```python
from build123d import *

# Parameters (mm, degrees)
SKETCH_1_W          = 260
SKETCH_1_H          = 236
EXTRUDE_1_DEPTH     = 3
SKETCH_2_R          = 2.25
SKETCH_2_R_2        = 3.5
CUT_EXTRUDE_1_DEPTH = 4
SKETCH1_R           = 2.25
CUT_EXTRUDE1_DEPTH  = 4


with BuildPart() as part:
    # Эскиз1 → Бобышка-Вытянуть1 (new body)
    with BuildSketch(Plane.XZ):
        with Locations((-88.97919902, 98.072268451)):
            Rectangle(SKETCH_1_W, SKETCH_1_H)
    extrude(amount=EXTRUDE_1_DEPTH)

    # Эскиз2 → Вырез-Вытянуть1 (cut, through all)
    with BuildSketch(Plane.XZ.offset(3)):
        with Locations((-208.97919902, 98.072268451)):
            Circle(SKETCH_2_R)
        with Locations((-148.97919902, -9.927731549)):
            Circle(SKETCH_2_R)
        with Locations((-28.97919902, -9.927731549)):
            Circle(SKETCH_2_R)
        with Locations((31.02080098, 98.072268451)):
            Circle(SKETCH_2_R)
        with Locations((-28.97919902, 206.072268451)):
            Circle(SKETCH_2_R)
        with Locations((-148.97919902, 206.072268451)):
            Circle(SKETCH_2_R)
        with Locations((-208.97919902, -9.927731549)):
            Circle(SKETCH_2_R_2)
        with Locations((-208.97919902, 206.072268451)):
            Circle(SKETCH_2_R_2)
        with Locations((31.02080098, -9.927731549)):
            Circle(SKETCH_2_R_2)
        with Locations((31.02080098, 206.072268451)):
            Circle(SKETCH_2_R_2)
    extrude(amount=-CUT_EXTRUDE_1_DEPTH, mode=Mode.SUBTRACT)

    # Sketch1 → Cut-Extrude1 (cut, through all)
    with BuildSketch(Plane(origin=(0, 0, 0), x_dir=(1, 0, 0), z_dir=(0, 1, 0))):
        with Locations((-31.97919902, -141.072268451)):
            Circle(SKETCH1_R)
        with Locations((11.02080098, -98.072268451)):
            Circle(SKETCH1_R)
        with Locations((-31.97919902, -55.072268451)):
            Circle(SKETCH1_R)
    extrude(amount=-CUT_EXTRUDE1_DEPTH, mode=Mode.SUBTRACT)


solid = part.part
```
Check sheet for the modelled part. Datum: model origin and axes. Units: mm. Give positions to 0.01 mm unless a question says otherwise; leave off trailing zeros. Answer as CSV lines item,"result".
Item 1: Scan lines: L1, parallel to Z at x = -30, y = -1.05; L2, parallel to X at y = -2.4, z = 203.5; L3, parallel to X at y = -1.9, z = 99. Record each from-to range of solid material in increasing order.
Reply:
L1,"-19.93 to -11.93, -7.92 to 54, 56.14 to 140, 142.14 to 204.07, 208.08 to 216.07"
L2,"-218.98 to -211.35, -206.61 to 28.65, 33.39 to 41.02"
L3,"-218.98 to -211.03, -206.93 to 8.97, 13.07 to 28.97, 33.07 to 41.02"
Item 2: Depth check by flat-ended pin: pin 1 Ø4 at (x, z) = (-148.98, 206.07) entering from -Y; pin 2 Ø6 at (x, z) = (-28.98, -9.93) entering from -Y. Enter the tip coordinate at first touch or a pass-through.
Reply:
pin 1,"through"
pin 2,"y = -3"
Item 3: Draft check along Z on faces 1 (the face through (-91, -3, 100)), 2 (the face through (27.524, -1.521, -9.774)). Enter one of: pulls with the +Z half, pulls with the -Z half, needs draft (parallel to the pull), parting line crosses it, or undercut.
Reply:
face 1,"needs draft"
face 2,"undercut"
